```python
from build123d import *

# Parameters (mm, degrees)
BOSS_EXTRUDE1_DEPTH      = 2
FILLET1_R                = 2
BOSS_EXTRUDE2_DEPTH      = 3
BOSS_EXTRUDE2_DEPTH_BACK = 2
SKETCH2_R                = 3.5
SKETCH3_R                = 2.5
CUT_EXTRUDE1_DEPTH       = 1
SKETCH4_R                = 1
CUT_EXTRUDE2_DEPTH       = 17.8597153
CUT_EXTRUDE3_START       = -3
SKETCH5_R                = 2.5
CUT_EXTRUDE3_DEPTH       = 3
CUT_EXTRUDE4_DEPTH       = 3
CIRPATTERN1_COUNT        = 36
SKETCH9_R                = 0.5
CUT_EXTRUDE5_DEPTH       = 18.12454379
LPATTERN1_COUNT          = 6
LPATTERN1_PITCH          = 2
MIRROR1_COPY_1_SKETCH_R  = 0.5
MIRROR1_COPY_1_DEPTH     = 18.12454379
MIRROR1_COPY_2_SKETCH_R  = 0.5
MIRROR1_COPY_2_DEPTH     = 18.12454379
MIRROR1_COPY_3_SKETCH_R  = 0.5
MIRROR1_COPY_3_DEPTH     = 18.12454379
MIRROR1_COPY_4_SKETCH_R  = 0.5
MIRROR1_COPY_4_DEPTH     = 18.12454379
MIRROR1_COPY_5_SKETCH_R  = 0.5
MIRROR1_COPY_5_DEPTH     = 18.12454379
FILLET3_R                = 2


with BuildPart() as part:
    # Sketch1 → Boss-Extrude1 (new body)
    with BuildSketch(Plane(origin=(0, 0, 0), x_dir=(1, 0, 0), z_dir=(0, 1, 0))):
        Polygon((-3.25, -1.75), (-3.25, 1.75), (-2, 16), (2, 16), (3.25, 1.75), (3.25, -1.75), (2, -16), (-2, -16), align=None)
    extrude(amount=BOSS_EXTRUDE1_DEPTH)

    # Fillet1
    fillet1_edges = [part.edges().sort_by_distance(p)[0] for p in [
        (-2, 1, -16),
        (2, 1, -16),
        (2, 1, 16),
        (-2, 1, 16),
    ]]
    fillet(fillet1_edges, radius=FILLET1_R)

    # Sketch2 → Boss-Extrude2 (add, two sides: drawn at the far end of the back side and taken through both)
    with BuildSketch(Plane(origin=(0, 2, 0), x_dir=(1, 0, 0), z_dir=(0, 1, 0)).offset(-BOSS_EXTRUDE2_DEPTH_BACK)):
        with Locations(Location((0, 0, 0), (0, 0, 270))):
            Circle(SKETCH2_R)
    extrude(amount=BOSS_EXTRUDE2_DEPTH + BOSS_EXTRUDE2_DEPTH_BACK)

    # Sketch3 → Cut-Extrude1 (cut)
    with BuildSketch(Plane(origin=(0, 0, 0), x_dir=(-1, 0, 0), z_dir=(0, -1, 0))):
        with Locations(Location((0, 0, 0), (0, 0, 90))):
            Circle(SKETCH3_R)
    extrude(amount=-CUT_EXTRUDE1_DEPTH, mode=Mode.SUBTRACT)

    # Sketch4 → Cut-Extrude2 (cut, through all)
    with BuildSketch(Plane(origin=(0, 1, 0), x_dir=(-1, 0, 0), z_dir=(0, -1, 0))):
        with Locations(Location((0, 0, 0), (0, 0, 90))):
            Circle(SKETCH4_R)
    extrude(amount=-CUT_EXTRUDE2_DEPTH, mode=Mode.SUBTRACT)

    # Sketch5 → Cut-Extrude3 (cut)
    with BuildSketch(Plane(origin=(0, 5, 0), x_dir=(1, 0, 0), z_dir=(0, 1, 0)).offset(CUT_EXTRUDE3_START)):
        with Locations(Location((0, 0, 0), (0, 0, 90))):
            Circle(SKETCH5_R)
    extrude(amount=CUT_EXTRUDE3_DEPTH, mode=Mode.SUBTRACT)

    # Sketch6 → Cut-Extrude4 (cut)
    with BuildSketch(Plane(origin=(0, 5, 0), x_dir=(1, 0, 0), z_dir=(0, 1, 0))):
        Polygon((-2.5, 0), (-2.691676801, 0.211839558), (-2.469220851, 0.391086163), align=None)
    cut_extrude4 = extrude(amount=-CUT_EXTRUDE4_DEPTH, mode=Mode.SUBTRACT)

    # CirPattern1: Cut-Extrude4 ×36 about axis
    cirpattern1_axis = Axis((0, 0, 0), (0, 1, 0))
    for i in range(1, CIRPATTERN1_COUNT):
        add(cut_extrude4.rotate(cirpattern1_axis, i * 360 / CIRPATTERN1_COUNT), mode=Mode.SUBTRACT)

    # Sketch9 → Cut-Extrude5 (cut, through all)
    with BuildSketch(Plane(origin=(0, 0, 0), x_dir=(-1, 0, 0), z_dir=(0, -1, 0))):
        with Locations(Location((0, 14.5, 0), (0, 0, 90))):
            Circle(SKETCH9_R)
    cut_extrude5 = extrude(amount=-CUT_EXTRUDE5_DEPTH, mode=Mode.SUBTRACT)

    # LPattern1: Cut-Extrude5 ×6
    with Locations(*[(0, 0, i * LPATTERN1_PITCH) for i in range(1, LPATTERN1_COUNT)]):
        add(cut_extrude5, mode=Mode.SUBTRACT)

    # Mirror1: Cut-Extrude5 across plane
    add(cut_extrude5.mirror(Plane.XY), mode=Mode.SUBTRACT)

    # Mirror1 copy 1 sketch → Mirror1 copy 1 (cut, through all)
    with BuildSketch(Plane(origin=(0, 0, -2), x_dir=(-1, 0, 0), z_dir=(0, -1, 0))):
        with Locations((0, -14.5)):
            Circle(MIRROR1_COPY_1_SKETCH_R)
    extrude(amount=-MIRROR1_COPY_1_DEPTH, mode=Mode.SUBTRACT)

    # Mirror1 copy 2 sketch → Mirror1 copy 2 (cut, through all)
    with BuildSketch(Plane(origin=(0, 0, -4), x_dir=(-1, 0, 0), z_dir=(0, -1, 0))):
        with Locations((0, -14.5)):
            Circle(MIRROR1_COPY_2_SKETCH_R)
    extrude(amount=-MIRROR1_COPY_2_DEPTH, mode=Mode.SUBTRACT)

    # Mirror1 copy 3 sketch → Mirror1 copy 3 (cut, through all)
    with BuildSketch(Plane(origin=(0, 0, -6), x_dir=(-1, 0, 0), z_dir=(0, -1, 0))):
        with Locations((0, -14.5)):
            Circle(MIRROR1_COPY_3_SKETCH_R)
    extrude(amount=-MIRROR1_COPY_3_DEPTH, mode=Mode.SUBTRACT)

    # Mirror1 copy 4 sketch → Mirror1 copy 4 (cut, through all)
    with BuildSketch(Plane(origin=(0, 0, -8), x_dir=(-1, 0, 0), z_dir=(0, -1, 0))):
        with Locations((0, -14.5)):
            Circle(MIRROR1_COPY_4_SKETCH_R)
    extrude(amount=-MIRROR1_COPY_4_DEPTH, mode=Mode.SUBTRACT)

    # Mirror1 copy 5 sketch → Mirror1 copy 5 (cut, through all)
    with BuildSketch(Plane(origin=(0, 0, -10), x_dir=(-1, 0, 0), z_dir=(0, -1, 0))):
        with Locations((0, -14.5)):
            Circle(MIRROR1_COPY_5_SKETCH_R)
    extrude(amount=-MIRROR1_COPY_5_DEPTH, mode=Mode.SUBTRACT)

    # Fillet3
    # the kernel refuses this fillet: 2 mm, written as the material it adds along each edge
    with BuildSketch(Plane(origin=(-3.25, 0, 1.299038106), x_dir=(-0.33486149994796977, 0, -0.9422673590083633), z_dir=(0, 1, 0))) as fillet3_piece_1:
        with BuildLine():
            CenterArc((0.349049135, 1.998495294), FILLET3_R, 250.435883949, 17.341442803)
            Line((-0.320673865, 0.113960576), (0, 0))
            ThreePointArc((0, 0), (0.13574133, 0.002633235), (0.271482661, 0))
        make_face()
    extrude(amount=2)
    with BuildSketch(Plane(origin=(3.25, 0, 1.299038106), x_dir=(0.3348614999479675, 0, -0.942267359008364), z_dir=(0, 1, 0))) as fillet3_piece_2:
        with BuildLine():
            CenterArc((0.349049135, -1.998495294), FILLET3_R, 92.222673248, 17.341442803)
            Line((-0.320673865, -0.113960576), (0, 0))
            ThreePointArc((0, 0), (0.13574133, -0.002633235), (0.271482661, 0))
        make_face()
    extrude(amount=2)
    with BuildSketch(Plane(origin=(-3.25, 0, -1.299038106), x_dir=(0, 0, -1), z_dir=(0, 1, 0))) as fillet3_piece_3:
        with BuildLine():
            CenterArc((0.340321525, 2), FILLET3_R, 252.658557197, 17.341442803)
            ThreePointArc((-0.25580925, 0.090909091), (-0.127022856, 0.047935757), (0, 0))
            Line((0, 0), (0.340321525, 0))
        make_face()
    extrude(amount=2)
    with BuildSketch(Plane(origin=(3.25, 0, -1.299038106), x_dir=(0, 0, -1), z_dir=(0, 1, 0))) as fillet3_piece_4:
        with BuildLine():
            CenterArc((0.340321525, -2), FILLET3_R, 90, 17.341442803)
            ThreePointArc((-0.25580925, -0.090909091), (-0.127022856, -0.047935757), (0, 0))
            Line((0, 0), (0.340321525, 0))
        make_face()
    extrude(amount=2)
    # the kernel refuses this fillet: 2 mm, written as the material it takes off along each edge
    with BuildSketch(Plane(origin=(3.25, -0.218878004, -1.75), x_dir=(0, 0, 1), z_dir=(0, 1, 0)), Plane(origin=(3.25, -0.218878004, 1.75), x_dir=(-0.08738374771484606, 0, 0.9961747239492218), z_dir=(0, 1, 0)), Plane(origin=(-3.25, -0.218878004, -1.75), x_dir=(0.08738374771484518, 0, -0.9961747239492218), z_dir=(0, 1, 0))) as fillet3_2_piece_1:
        with BuildLine():
            CenterArc((FILLET3_R * 0.043775600736, -FILLET3_R), FILLET3_R, 90, 5.013113755)
            Line((-FILLET3_R * 0.0436081469789, -FILLET3_R * 0.00382527605078), (0, 0))
            Line((0, 0), (FILLET3_R * 0.043775600736, 0))
        make_face()
    extrude(amount=2.437756007, mode=Mode.SUBTRACT)
    with BuildSketch(Plane(origin=(-3.25, -0.218878004, 1.75), x_dir=(0.08738374771484235, 0, 0.996174723949222), z_dir=(0, 1, 0))) as fillet3_2_piece_2:
        with BuildLine():
            CenterArc((FILLET3_R * 0.043775600736, FILLET3_R), FILLET3_R, 264.986886245, 5.013113755)
            Line((-FILLET3_R * 0.0436081469789, FILLET3_R * 0.00382527605078), (0, 0))
            Line((0, 0), (FILLET3_R * 0.043775600736, 0))
        make_face()
    extrude(amount=2.437756007, mode=Mode.SUBTRACT)


solid = part.part
```
Build history of the part. All positions in model axes, mm. A direction names the side the tool comes from. Give positions to 0.01 mm unless a question says otherwise; leave off trailing zeros. Loops run counter-clockwise (first coordinate to the right, second up) from the corner with the lowest first, then second, coordinate; pieces in that order, holes last. Notation, with made-up numbers: (-32, 85.5) -> (-17, 85.5) arc R33 ccw to (-17, 123.5) -> close; hole circle Ø8 at (73.5, -34). An arc over 180 degrees is marked (long way). One line per question, with ' | ' between items. Start each with the question number.
1) Cut at A-A (z = 4.5). Give the cut face in (x, y), plus the area to 3 significant figures.
2) Pin check, flat tips, straight feed: pin 1 (2.5 mm diameter, centred on x = 0, z = 0, fed in from +Y); pin 2 (3 mm diameter, centred on y = 3, z = 5, fed in from -X); pin 3 (1.5 mm diameter, centred on x = 1, z = 1, fed in from -Y). Stop position of each tip, or through.
3) Two-plate mould, pull along X, no slides. Class faces 1 (the cylindrical face through (1.534, 1.014, 15.461)), 2 (the flat face through (3, 0, 0)), 3 (the cylindrical face through (0, 1, -13)): released by +X, released by -X, zero draft, split by the parting line, or undercut.
4) Probe L1, parallel to Y at x = -1.5, z = 12; L2, parallel to X at y = 0.95, z = 8.5; L3, parallel to X at y = 1.55, z = -6.5. List the from-to ranges inside material, lowest first.
5) Cut at B-B (z = -10.5). Give the cut face in (x, y).
6) 3-axis set-ups, long thin cutter, end or side, ignore diameter. For faces 4 (the cylindrical face through (1.5, 1.01, -15.49)), 5 (the flat face through (-1, 1, -1)), 6 (the cylindrical face through (0.154, 3.021, -3.497)): which of +Z, -Z, +X, -X, +Y, -Y reach the whole face in a straight line?
Return value:
1) outline: (-3.01, 0) -> (-0.5, 0) -> (-0.5, 2) -> (-3.01, 2) -> close; (0.5, 0) -> (3.01, 0) -> (3.01, 2) -> (0.5, 2) -> close | area: 10.0 mm^2
2) pin 1: y = 2 | pin 2: x = -3.06 | pin 3: y = 1
3) face 1: released by +X | face 2: zero draft | face 3: undercut
4) L1: 0 to 2 | L2: -2.66 to -0.5, 0.5 to 2.66 | L3: -2.83 to -0.5, 0.5 to 2.83
5) outline: (-2.48, 0) -> (-0.5, 0) -> (-0.5, 2) -> (-2.48, 2) -> close; (0.5, 0) -> (2.48, 0) -> (2.48, 2) -> (0.5, 2) -> close
6) face 4: -Z, +X, +Y, -Y | face 5: -Y | face 6: +Y
